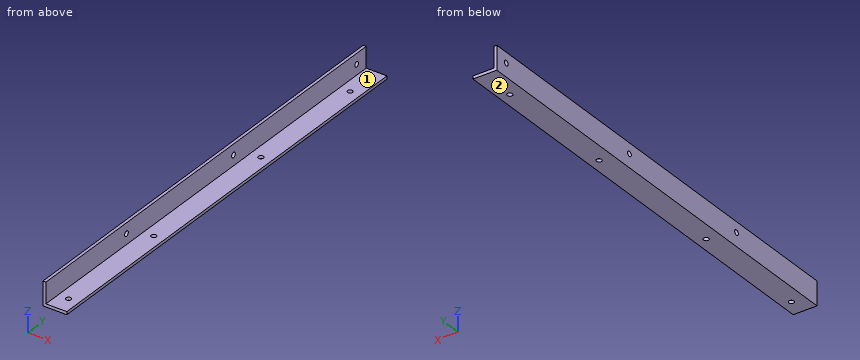
Autodesk Fusion 360 part; units mm, degrees
sketch "Sketch1" plane through (0, 0, 0) normal (0, 1, 0) x (1, 0, 0)
  line L0 (0, 0) -> (25.4, 0)
  line L1 (25.4, 0) -> (25.4, -3.175)
  line L2 (25.4, -3.175) -> (3.175, -3.175)
  line L3 (3.175, -3.175) -> (3.175, -25.4)
  line L4 (3.175, -25.4) -> (0, -25.4)
  line L5 (0, -25.4) -> (0, 0)
  dimension "d1" = 25.4
  dimension "d2" = 25.4
  dimension "d3" = 3.175
  dimension "d4" = 3.175
extrude "Extrude1" add sketch "Sketch1" along normal blind 480
sketch "Sketch2" plane through (0, 0, 3.175) normal (0, 0, 1) x (1, 0, 0)
  line L0 (3.175, 0) -> (25.4, 0)
  line L1 (25.4, 0) -> (25.4, 480)
  line L2 (25.4, 480) -> (3.175, 480)
  line L3 (3.175, 480) -> (3.175, 0)
  circle A0 centre (14.2875, 18.25) radius 2.75
  circle A1 centre (14.2875, 146.11) radius 2.75
  circle A2 centre (14.2875, 306.51) radius 2.75
  circle A3 centre (14.2875, 440.31) radius 2.75
  line L4 (14.2875, 480) -> (14.2875, 0) construction
  dimension "d7" = 18.25
  dimension "d8" = 146.11
  dimension "d9" = 306.51
  dimension "d10" = 440.31
  dimension "d11" = 5.5
sketch "Sketch3" plane through (3.175, 0, 0) normal (1, 0, 0) x (0, 0, -1)
  line L0 (-25.4, 0) -> (-3.175, 0)
  line L1 (-3.175, 0) -> (-3.175, 480)
  line L2 (-3.175, 480) -> (-25.4, 480)
  line L3 (-25.4, 480) -> (-25.4, 0)
  circle A0 centre (-14.2875, 120.71) radius 2.75
  circle A1 centre (-14.2875, 281.11) radius 2.75
  circle A2 centre (-14.2875, 465.71) radius 2.75
  line L4 (-14.2875, 480) -> (-14.2875, 0) construction
  dimension "d12" = 120.71
  dimension "d13" = 5.5
  dimension "d14" = 281.11
  dimension "d15" = 465.71
hole "Hole1" at (3.175, 465.71, 14.2875) at (3.175, 281.11, 14.2875) at (3.175, 120.71, 14.2875) direction (-1, 0, 0) diameter 5.5 depth 7 tip angle 118
hole "Hole2" at (14.2875, 440.31, 3.175) at (14.2875, 306.51, 3.175) at (14.2875, 146.11, 3.175) at (14.2875, 18.25, 3.175) direction (0, 0, -1) diameter 5.5 depth 7 tip angle 118
equation "d3 = ( 1 / 8 ) * 1 in"
equation "d4 = ( 1 / 8 ) * 1 in"
equation "d8 = 135 mm + 11.11 mm"
equation "d9 = 295.4 mm + 11.11 mm"
equation "d10 = 429.2 mm + 11.11 mm"
equation "d12 = 109.6 mm + 11.11 mm"
equation "d14 = 270 mm + 11.11 mm"
equation "d15 = 454.6 mm + 11.11 mm"
Can you work these out from the model? Positions are in its coordinate system, mm. Face numbers are marked on the shaded views. A direction names the side the tool comes from. Coordinates: 2 decimals unless noted, no trailing zeros. Order: outer loops, then holes, each group sorted by start corner. A loop starts at its lowest first (then second) coordinate and runs counter-clockwise, first axis right, second up. Notation, with made-up numbers: (20, -13.75) -> (50, -13.75) arc R14 ccw to (50, 11.25) -> close; hole circle Ø6 at (11, 33). An arc over 180 degrees is marked (long way). Use one line per item in the form item = value.
Q1. I need wall thicknesses on L1, parallel to X at y = 146.11, z = 1.95; L2, parallel to Z at x = 9.25, y = 241 (3 decimals). Which ranges of each line are inside material? Lowest first, please.
From the geometry:
L1 = 0 to 11.54, 17.04 to 25.4
L2 = 0 to 3.175
Q2. Will these pins go through, and if not, where does the flat tip stop? P1, Ø7, axis at x = 14.29, y = 146.11, coming from the +Z side (3 decimals); P2, Ø3, axis at y = 72, z = 5.5, coming from the +X side (3 decimals); P3, Ø5, axis at x = 14.29, y = 306.51, coming from the +Z side.
From the geometry:
P1 = 3.175
P2 = 3.175
P3 = through
Q3. Imagine slicing it at A-A, the plane y = 162.5. List the corners of the cut face in (x, z) for me (3 decimals).
From the geometry:
outline = (0, 0) -> (25.4, 0) -> (25.4, 3.175) -> (3.175, 3.175) -> (3.175, 25.4) -> (0, 25.4) -> close
Q4. Which directions (+Z, -Z, +X, -X, +Y, -Y) give clear straight access to the entire face, cutting with the end or side of a thin tool? Please do the marked faces 1 and 2.
From the geometry:
face_1 = +Z, +X, +Y, -Y
face_2 = -Z, +X, -X, +Y, -Y
